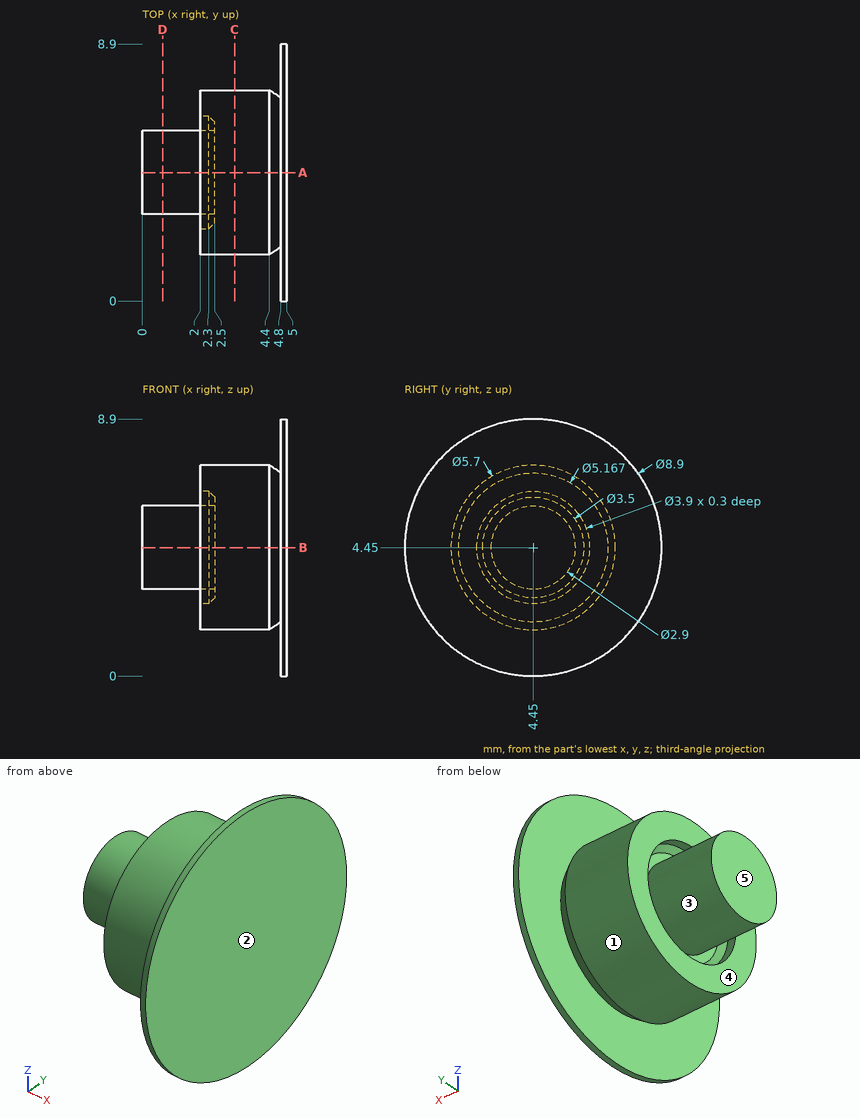
Design review of the part shown in the three views and the two pictorial views. Dimensions are in mm from the part's minimum x, y and z. A direction names the side the tool comes from. Coordinates: 2 decimals unless noted, no trailing zeros. Write each loop counter-clockwise with the first axis right and the second up, starting at its lowest first coordinate (ties: lowest second). Pieces come first, ordered by that corner, then holes.
1) We need section A-A on y = 4.45. State the section outline as (x, z) points, then the cut area to 3 significant figures.
2) To check wall thickness, follow probe 1 along Z at (x, y) = (2.25, 4.45); probe 2 along Z at (x, y) = (2.2, 4) (1 decimal); probe 3 along X at (y, z) = (6, 3). State the ranges of each line that lie inside material, in increasing order.
3) We need section C-C on x = 3.2. State the section outline as (y, z) points.
4) The part is to be moulded in two halves that separate along Z. For the marked faces 1, 2 and 3, say which applies: pulls with the +Z half, pulls with the -Z half, needs draft (parallel to the pull), parting line crosses it, or undercut.
5) We need section D-D on x = 0.7. State the section outline as (y, z) points.
6) Machinability: for the marked faces 4 and 5, which of the approach directions +Z, -Z, +X, -X, +Y, -Y give a long, thin tool a straight path to every point of the face, cutting with its end or side? Answer none if there is none.
7) Clearance check with flat-ended pins moving along their axes: pin 1 Ø2 at (x, z) = (0.5, 6.5) entering from +Y; pin 2 Ø2 at (x, z) = (4, 6.5) entering from +Y; pin 3 Ø1.5 at (x, z) = (2.5, 6) entering from -Y (1 decimal). State where each tip first meets the part, or that it passes through.
Answer list:
1. outline: (0, 3) - (2.5, 3) - (2.5, 2.7) - (2.3, 2.5) - (2, 2.5) - (2, 1.6) - (4.4, 1.6) - (4.8, 1.87) - (4.8, 0) - (5, 0) - (5, 8.9) - (4.8, 8.9) - (4.8, 7.03) - (4.4, 7.3) - (2, 7.3) - (2, 6.4) - (2.3, 6.4) - (2.5, 6.2) - (2.5, 5.9) - (0, 5.9) - close
1. area: 23.0 mm2
2. probe 1: z = 1.6 to 2.5, 3 to 5.9, 6.4 to 7.3
2. probe 2: z = 1.6 to 2.6, 3.1 to 5.8, 6.3 to 7.3
2. probe 3: x = 2 to 5
3. outline: circle Ø5.7 at (4.45, 4.45)
4. face 1: parting line crosses it
4. face 2: needs draft
4. face 3: undercut
5. outline: circle Ø2.9 at (4.45, 4.45)
6. face 4: -X
6. face 5: +Z, -Z, -X, +Y, -Y
7. pin 1: stops at y = 5.45
7. pin 2: stops at y = 8.66
7. pin 3: stops at y = 1.7
